```python
from build123d import *

# Parameters (mm, degrees)
SKETCH1_R           = 6.35
SKETCH1_R_2         = 5.08
BOSS_EXTRUDE1_DEPTH = 26.035
SKETCH2_R           = 20.6375
BOSS_EXTRUDE2_DEPTH = 6.35
SKETCH3_R           = 5.08
BOSS_EXTRUDE3_DEPTH = 15.875


with BuildPart() as part:
    # Sketch1 → Boss-Extrude1 (new body)
    with BuildSketch(Plane(origin=(0, 0, 0), x_dir=(1, 0, 0), z_dir=(0, 1, 0))):
        with Locations(Location((0, 0, 0), (0, 0, 270))):
            Circle(SKETCH1_R)
        with Locations(Location((0, 0, 0), (0, 0, 270))):
            Circle(SKETCH1_R_2, mode=Mode.SUBTRACT)
    extrude(amount=BOSS_EXTRUDE1_DEPTH)

    # Sketch2 → Boss-Extrude2 (add)
    with BuildSketch(Plane.XZ):
        with Locations(Location((0, 0, 0), (0, 0, 270))):
            Circle(SKETCH2_R)
    extrude(amount=BOSS_EXTRUDE2_DEPTH)

    # Sketch3 → Boss-Extrude3 (add)
    with BuildSketch(Plane(origin=(0, 0, 0), x_dir=(1, 0, 0), z_dir=(0, 1, 0))):
        with Locations(Location((0, 0, 0), (0, 0, 270))):
            Circle(SKETCH3_R)
    extrude(amount=BOSS_EXTRUDE3_DEPTH)


solid = part.part
```
Read the model definition and answer for the solid it produces. Units are mm, in the model's axes. A direction names the side the tool comes from. Give positions to 0.01 mm unless a question says otherwise; leave off trailing zeros. Write each loop counter-clockwise with the first axis right and the second up, starting at its lowest first coordinate (ties: lowest second). Pieces come first, ordered by that corner, then holes. Notation, with made-up numbers: M -25,39.5 L -5,39.5 A27 ccw -5,62.5 Z; hole C 28.5,52.25 d1. An arc over 180 degrees is marked long. Put each result on its own line as item: value. Start each with the question number.
1. Each of these flat-tipped pins is pushed along its axis until it touches: pin 1 Ø4 at (x, y) = (-6, 4.5) entering from -Z; pin 2 Ø1.5 at (y, z) = (13, 9) entering from -X; pin 3 Ø12 at (x, z) = (12, -8.5) entering from +Y; pin 4 Ø9 at (x, z) = (0, 0) entering from +Y (3 decimals). Where does it stop, or does it pass through?
2. Consider line 1 along X through (y, z) = (19.5, 0); line 2 along Y through (x, z) = (8, 2); line 3 along Z through (x, y) = (-4, 21.5). Determine where each line is inside the solid, lowest interval first.
3. The part is cut by section D-D, the plane y = 11.5. Give the vertices of the cut face in (x, z).
4. Which of the six approach directions +Z, -Z, +X, -X, +Y, -Y give full straight-line access (tool end or side, diameter ignored) to faces 5 (the flat face through (5, 26.035, 2)), 6 (the flat face through (-4.3, 0, 4.9))?
5. The part is cut by section C-C, the plane y = 22. Give the vertices of the cut face in (x, z).
6. For a pull along Z with two mould halves and no side action, classify faces 1 (the flat face through (0, 15.875, 0)), 2 (the cylindrical face through (-3.86, 12.84, -5.04)), 3 (the flat face through (0, -6.35, 0)), 4 (the cylindrical face through (5.037, 20.884, -0.661)) as released by +Z, released by -Z, zero draft, split by the parting line, or undercut.
Final values:
1. pin 1: stops at z = -4.93
1. pin 2: passes through
1. pin 3: stops at y = 0
1. pin 4: stops at y = 15.875
2. line 1: x = -6.35 to -5.08, 5.08 to 6.35
2. line 2: y = -6.35 to 0
2. line 3: z = -4.93 to -3.13, 3.13 to 4.93
3. outline: C 0,0 d12.7
4. face 5: +Z, -Z, +X, -X, +Y
4. face 6: +Y
5. outline: C 0,0 d12.7; hole C 0,0 d10.16
6. face 1: undercut
6. face 2: split by the parting line
6. face 3: zero draft
6. face 4: undercut
